Read the model definition and answer for the solid it produces. Units are mm, in the model's axes. A direction names the side the tool comes from. Coordinates: 2 decimals unless noted, no trailing zeros. Loops run counter-clockwise (first coordinate to the right, second up) from the corner with the lowest first, then second, coordinate; pieces in that order, holes last. Notation, with made-up numbers: M -25,62 L 32,62 A20 cw 32,91 Z; hole C -2,45.25 d2. An arc over 180 degrees is marked long. Use one line per item in the form item = value. Start each with the question number.
1. A tool of negligible diameter and unlimited length cuts with its end or side. For faces 4 (the flat face through (28, 16.671, 2)), 5 (the cylindrical face through (48.416, 0.781, 2.028)), from which of +Z, -Z, +X, -X, +Y, -Y can it reach the whole face along a straight path? Write none if from no direction.
2. The part is cut by section D-D (y = 0.5). Give the number of separate pieces and of enclosed holes in the cut face, plus the area to 3 significant figures.
3. The part is cut by section A-A (x = 38). Give the vertices of the cut face in (y, z).
4. The part is cut by section C-C (x = 9.5). Give the vertices of the cut face in (y, z), plus the area to 3 significant figures.
5. Flat-ended cylindrical pins translate along their axes: pin 1 (5 mm diameter, centred on x = 23, y = 12, fed in from -Z); pin 2 (6.5 mm diameter, centred on x = -3.88, y = 0.67, fed in from +Z); pin 3 (8 mm diameter, centred on x = 60.72, y = 0.67, fed in from +Z). Find the tip coordinate at first contact, or state that the pin passes through.
6. The part is cut by section B-B (z = 2.1). Give the vertices of the cut face in (x, y), plus the area to 3 significant figures.
7. Find the intervals of material crossed by probe 1 along Y at (x, z) = (15, 1.5); probe 2 along X at (y, z) = (3, 0.2); probe 3 along X at (y, z) = (1.5, 3.2), in increasing order. Write a range as [from, to].
8. For a pull along X with two mould halves and no side action, classify faces 1 (the flat face through (-19.882, 0, 2)), 2 (the flat face through (29, -4.329, 2)), 3 (the flat face through (76.718, 0, 2)) as released by +X, released by -X, zero draft, split by the parting line, or undercut.
from build123d import *

# Parameters (mm, degrees)
SKETCH1_W                                  = 96.6
SKETCH1_H                                  = 32
BOSS_EXTRUDE1_DEPTH                        = 4
CUT_EXTRUDE1_DEPTH                         = 5
FRAISAGE_POUR_VIS_T_TE_FRAIS_E_BOM_2_COUNT = 2
FRAISAGE_POUR_VIS_T_TE_FRAIS_E_BOM_2_PITCH = 64.6


with BuildPart() as part:
    # Sketch1 → Boss-Extrude1 (new body)
    with BuildSketch(Plane.XY):
        with Locations((28.417538555, 0.671328671)):
            Rectangle(SKETCH1_W, SKETCH1_H)
    extrude(amount=BOSS_EXTRUDE1_DEPTH)

    # Sketch2 → Cut-Extrude1 (cut, through all)
    with BuildSketch(Plane.XY.offset(4)):
        with BuildLine():
            Line((13.417538555, 5.671328671), (43.417538555, 5.671328671))
            ThreePointArc((43.417538555, 5.671328671), (48.417538555, 0.671328671), (43.417538555, -4.328671329))
            Line((43.417538555, -4.328671329), (13.417538555, -4.328671329))
            ThreePointArc((13.417538555, -4.328671329), (8.417538555, 0.671328671), (13.417538555, 5.671328671))
        make_face()
    extrude(amount=-CUT_EXTRUDE1_DEPTH, mode=Mode.SUBTRACT)

    # Esquisse3 → Fraisage pour vis à tête fraisée bombée #51 (revolve, cut)
    with BuildSketch(Plane(origin=(-3.882461445, 0.671328671, 4), x_dir=(0, -1, 0), z_dir=(1, 0, 0))):
        Polygon((0, 0), (0, 4), (2.54999998, 4), (2.54999998, 2.700000061), (5.250000041, 0), align=None)
    fraisage_pour_vis_t_te_frais_e_bomb_e = revolve(axis=Axis((-3.882461445, 0.671328671, 10.35), (0, 0, -1)), mode=Mode.SUBTRACT)

    # Fraisage pour vis _ t_te frais_e bom 2: Fraisage pour vis à tête fraisée bombée #51 ×2
    with Locations(*[(i * FRAISAGE_POUR_VIS_T_TE_FRAIS_E_BOM_2_PITCH, 0, 0) for i in range(1, FRAISAGE_POUR_VIS_T_TE_FRAIS_E_BOM_2_COUNT)]):
        add(fraisage_pour_vis_t_te_frais_e_bomb_e, mode=Mode.SUBTRACT)


solid = part.part
Computed values:
q1.face_4 = +Z, -Z, +X, -X, +Y
q1.face_5 = +Z, -Z
q2.separate_pieces = 4
q2.enclosed_holes = 0
q2.area = 171 mm²
q3.outline = M -15.33,0 L -4.33,0 L -4.33,4 L -15.33,4 Z; M 5.67,0 L 16.67,0 L 16.67,4 L 5.67,4 Z
q4.outline = M -15.33,0 L -2.44,0 L -2.44,4 L -15.33,4 Z; M 3.78,0 L 16.67,0 L 16.67,4 L 3.78,4 Z
q4.area = 103 mm²
q5.pin_1 = 0
q5.pin_2 = 2
q5.pin_3 = 2.75
q6.outline = M -19.88,-15.33 L 76.72,-15.33 L 76.72,16.67 L -19.88,16.67 Z; hole C -3.88,0.67 d6.7; hole M 13.42,-4.33 L 43.42,-4.33 A5 ccw 43.42,5.67 L 13.42,5.67 A5 ccw Z; hole C 60.72,0.67 d6.7
q6.area = 2,640 mm²
q7.probe_1 = [-15.33, -4.33], [5.67, 16.67]
q7.probe_2 = [-19.88, -4.92], [-2.84, 8.99], [47.84, 59.68], [61.76, 76.72]
q7.probe_3 = [-19.88, -8.25], [0.49, 8.49], [48.35, 56.35], [65.09, 76.72]
q8.face_1 = released by -X
q8.face_2 = undercut
q8.face_3 = released by +X
